The model under review builds one solid part; all positions refer to its coordinate system, in mm. A direction names the side the tool comes from. Coordinates: 2 decimals unless noted, no trailing zeros. Write each loop counter-clockwise with the first axis right and the second up, starting at its lowest first coordinate (ties: lowest second). Pieces come first, ordered by that corner, then holes.
1) Mouldability with a two-part tool opening along Z and no side actions: class faces 1 (the flat face through (0, 21.2, 0)), 2 (the cylindrical face through (15.777, 16.27, -8.445)), 3 (the cylindrical face through (-23.64, 10.45, 12.3)) as released by +Z, released by -Z, zero draft, split by the parting line, or undercut.
2) Add section B-B, the plane z = -2. State the section outline as (x, y) points (1 decimal), then the cut area to 3 significant figures.
3) Add section A-A, the plane x = 0. State the section outline as (y, z) points, then the cut area to 3 significant figures.
4) For P1, Ø1, axis at x = 4, y = 10, coming from the +Z side; P2, Ø3, axis at y = 14.5, z = 16, coming from the +X side; P3, Ø2.5, axis at x = -6.31, z = 15.24, coming from the -Y side (3 decimals), all flat-tipped, find the tip position at first contact; note any pin that passes through.
5) Add section D-D, the plane z = -8. State the section outline as (x, y) points, then the cut area to 3 significant figures.
6) Machinability: for faces 4 (the flat face through (0, 11.2, 16)), 5 (the flat face through (0, 0, 0)), 6 (the flat face through (-10, 8.255, -13)), which of the approach directions +Z, -Z, +X, -X, +Y, -Y give a long, thin tool a straight path to every point of the face, cutting with its end or side? Answer none if there is none.
7) For line 1 (X direction, y = 18.5, z = -8); line 2 (X direction, y = 5.5, z = -1); line 3 (X direction, y = 7.25, z = -3), list the stretches that pass through material, from the lowest coordinate up.
8) Add section C-C, the plane y = 19. State the section outline as (x, z) points.
from build123d import *

# Parameters (mm, degrees)
SKETCH1_R           = 26.65
BOSS_EXTRUDE1_DEPTH = 21.2
SKETCH6_R           = 1.5
CUT_EXTRUDE2_DEPTH  = 8.255
SKETCH7_R           = 1.5
CUT_EXTRUDE3_DEPTH  = 10


with BuildPart() as part:
    # Sketch1 → Boss-Extrude1 (new body)
    with BuildSketch(Plane(origin=(0, 0, 0), x_dir=(1, 0, 0), z_dir=(0, 1, 0))):
        with Locations(Location((0, 0, 0), (0, 0, 270))):
            Circle(SKETCH1_R)
    extrude(amount=BOSS_EXTRUDE1_DEPTH)

    # Sketch6 → Cut-Extrude2 (cut)
    with BuildSketch(Plane(origin=(0, 0, 0), x_dir=(-1, 0, 0), z_dir=(0, -1, 0))):
        with Locations(Location((6.313805851, -15.242875716, 0), (0, 0, 90))):
            Circle(SKETCH6_R)
        with Locations(Location((-16.357620523, 2.153521596, 0), (0, 0, 90))):
            Circle(SKETCH6_R)
        with Locations(Location((10.043814672, 13.08935412, 0), (0, 0, 90))):
            Circle(SKETCH6_R)
    extrude(amount=-CUT_EXTRUDE2_DEPTH, mode=Mode.SUBTRACT)

    # Sketch7 → Cut-Extrude3 (cut)
    with BuildSketch(Plane(origin=(0, 21.2, 0), x_dir=(1, 0, 0), z_dir=(0, 1, 0))):
        with Locations(Location((0, -16.5, 0), (0, 0, 270))):
            Circle(SKETCH7_R)
        with Locations(Location((-14.289419162, 8.25, 0), (0, 0, 270))):
            Circle(SKETCH7_R)
        with Locations(Location((14.289419162, 8.25, 0), (0, 0, 270))):
            Circle(SKETCH7_R)
    extrude(amount=-CUT_EXTRUDE3_DEPTH, mode=Mode.SUBTRACT)


solid = part.part
Geometry results:
1. face 1: zero draft
1. face 2: undercut
1. face 3: split by the parting line
2. outline: (-26.6, 0) - (14.9, 0) - (14.9, 8.3) - (17.8, 8.3) - (17.8, 0) - (26.6, 0) - (26.6, 21.2) - (-26.6, 21.2) - close
2. area: 1,100 mm2
3. outline: (0, -26.65) - (21.2, -26.65) - (21.2, 15) - (11.2, 15) - (11.2, 18) - (21.2, 18) - (21.2, 26.65) - (0, 26.65) - close
3. area: 1,100 mm2
4. P1: stops at z = 26.42
4. P2: stops at x = 22.36
4. P3: stops at y = 8.255
5. outline: (-25.42, 0) - (25.42, 0) - (25.42, 21.2) - (15.77, 21.2) - (15.77, 11.2) - (12.81, 11.2) - (12.81, 21.2) - (-12.81, 21.2) - (-12.81, 11.2) - (-15.77, 11.2) - (-15.77, 21.2) - (-25.42, 21.2) - close
5. area: 1,020 mm2
6. face 4: +Y
6. face 5: +Z, -Z, +X, -X, -Y
6. face 6: -Y
7. line 1: x = -25.42 to -15.77, -12.81 to 12.81, 15.77 to 25.42
7. line 2: x = -26.63 to 15.4, 17.32 to 26.63
7. line 3: x = -26.48 to 15.12, 17.6 to 26.48
8. outline: circle Ø53.3 at (0, 0); hole circle Ø3 at (-14.29, -8.25); hole circle Ø3 at (0, 16.5); hole circle Ø3 at (14.29, -8.25)
